```python
from build123d import *

# Parameters (mm, degrees)
F0_R      = 8.763
F1_DEPTH  = 17.526
F2_R      = 99.06
F3_DEPTH  = 163.576
F4_R      = 76.2
F5_DEPTH  = 38.1
F6_R      = 39.6875
F7_DEPTH  = 41.402
F9_R      = 88.9
F10_DEPTH = 9.398


with BuildPart() as f1:
    # F0 (on Top) → F1 (new body)
    with BuildSketch(Plane.XY):
        with BuildLine():
            Line((87.3125, 100.0125), (-87.3125, 100.0125))
            ThreePointArc((-87.3125, 100.0125), (-96.292756, 96.292756), (-100.0125, 87.3125))
            Line((-100.0125, 87.3125), (-100.0125, -87.3125))
            ThreePointArc((-100.0125, -87.3125), (-96.292756, -96.292756), (-87.3125, -100.0125))
            Line((-87.3125, -100.0125), (87.3125, -100.0125))
            ThreePointArc((87.3125, -100.0125), (96.292756, -96.292756), (100.0125, -87.3125))
            Line((100.0125, -87.3125), (100.0125, 87.3125))
            ThreePointArc((100.0125, 87.3125), (96.292756, 96.292756), (87.3125, 100.0125))
        make_face()
        with Locations((-80.822305, -80.822305)):
            Circle(F0_R, mode=Mode.SUBTRACT)
        with Locations((80.822305, -80.822305)):
            Circle(F0_R, mode=Mode.SUBTRACT)
        with Locations((-80.822305, 80.822305)):
            Circle(F0_R, mode=Mode.SUBTRACT)
        with Locations((80.822305, 80.822305)):
            Circle(F0_R, mode=Mode.SUBTRACT)
    extrude(amount=F1_DEPTH)

    # F2 (on face) → F3 (join)
    with BuildSketch(Plane.XY.offset(17.526)):
        Circle(F2_R)
    extrude(amount=-F3_DEPTH)

    # F4 (on face) → F5 (join)
    with BuildSketch(Plane.XY.offset(17.526)):
        Circle(F4_R)
    extrude(amount=F5_DEPTH)

    # F6 (on face) → F7 (join)
    with BuildSketch(Plane.XY.offset(55.626)):
        Circle(F6_R)
    extrude(amount=F7_DEPTH)

    # F9 (on offset) → F10 (join, through all)
    with BuildSketch(Plane.XY.offset(106.426)):
        Circle(F9_R)
    extrude(amount=-F10_DEPTH)


solid = f1.part
```
For this review, take the finished solid that the model builds, in its own axes (mm). A direction names the side the tool comes from. Round coordinates to 2 decimals unless told otherwise and drop trailing zeros. Write each loop counter-clockwise with the first axis right and the second up, starting at its lowest first coordinate (ties: lowest second). Pieces come first, ordered by that corner, then holes. Notation, with made-up numbers: (52, -18.75) - (76, -18.75) arc R18 ccw to (76, 9.25) - close; hole circle Ø1 at (-23, 13). An arc over 180 degrees is marked (long way). Put each result on its own line as item: value.
Q1. Mouldability with a two-part tool opening along X and no side actions: class faces 5 (the face through (33, -33, 55.626)), 6 (the face through (-76.779, -88.597, 8.64)), 7 (the face through (96.193, -96.391, 8.64)) as released by +X, released by -X, zero draft, split by the parting line, or undercut.
Solved:
face 5: zero draft
face 6: undercut
face 7: released by +X
Q2. We need section B-B (x = 0). Give the boundary of the cut face in (y, z), and give its area (3 significant figures).
Solved:
outline: (-100.01, 0) - (-99.06, 0) - (-99.06, -146.05) - (99.06, -146.05) - (99.06, 0) - (100.01, 0) - (100.01, 17.53) - (76.2, 17.53) - (76.2, 55.63) - (39.69, 55.63) - (39.69, 97.03) - (88.9, 97.03) - (88.9, 106.43) - (-88.9, 106.43) - (-88.9, 97.03) - (-39.69, 97.03) - (-39.69, 55.63) - (-76.2, 55.63) - (-76.2, 17.53) - (-100.01, 17.53) - close
area: 43,200 mm2
Q3. Machinability: for faces 1 (the face through (84.795, 26.703, 101.793)), 2 (the face through (-97, -22, 0)), 3 (the face through (100.012, -1, 9)), 4 (the face through (43, 68, 17.526)), which of the approach directions +Z, -Z, +X, -X, +Y, -Y give a long, thin tool a straight path to every point of the face, cutting with its end or side? Answer none if there is none.
Solved:
face 1: +Z
face 2: -Z
face 3: +Z, -Z, +X, +Y, -Y
face 4: none
Q4. We need section D-D (z = 7). Give the boundary of the cut face in (x, y).
Solved:
outline: (-100.01, -87.31) arc R12.7 ccw to (-87.31, -100.01) - (87.31, -100.01) arc R12.7 ccw to (100.01, -87.31) - (100.01, 87.31) arc R12.7 ccw to (87.31, 100.01) - (-87.31, 100.01) arc R12.7 ccw to (-100.01, 87.31) - close; hole circle Ø17.53 at (-80.82, -80.82); hole circle Ø17.53 at (-80.82, 80.82); hole circle Ø17.53 at (80.82, -80.82); hole circle Ø17.53 at (80.82, 80.82)
Q5. We need section A-A (y = -51). Give the boundary of the cut face in (x, z), and give its area (3 significant figures).
Solved:
outline: (-100.01, 0) - (-84.92, 0) - (-84.92, -146.05) - (84.92, -146.05) - (84.92, 0) - (100.01, 0) - (100.01, 17.53) - (56.62, 17.53) - (56.62, 55.63) - (-56.62, 55.63) - (-56.62, 17.53) - (-100.01, 17.53) - close; (-72.82, 97.03) - (72.82, 97.03) - (72.82, 106.43) - (-72.82, 106.43) - close
area: 34,000 mm2
Q6. Insertion check: pin 1 Ø6 at (y, z) = (-40, -55) entering from +X; pin 2 Ø23 at (x, y) = (80.82, -80.82) entering from -Z; pin 3 Ø1.5 at (y, z) = (-65, -59) entering from -X. Each pin has a flat end and moves straight along its axis. Give the tip position at first contact, or say it passes through.
Solved:
pin 1: stops at x = 91.89
pin 2: stops at z = 0
pin 3: stops at x = -75.4
Q7. Wall thickness on probe 1 along Z at (x, y) = (-23, 40.5); probe 2 along Z at (x, y) = (-83.5, 24); probe 3 along Z at (x, y) = (-76.5, 73): over which ranges is each line inside the solid? List them lowest first.
Solved:
probe 1: z = -146.05 to 55.63, 97.03 to 106.43
probe 2: z = -146.05 to 17.53, 97.03 to 106.43
probe 3: z = 0 to 17.53
